```python
from build123d import *

# Parameters (mm, degrees)
PAD_DEPTH       = 10
SKETCH001_W     = 14
SKETCH001_H     = 120
POCKET_DEPTH    = 2
SKETCH002_W     = 8
SKETCH002_H     = 112
POCKET001_DEPTH = 5
SKETCH003_W     = 23
SKETCH003_H     = 6
POCKET002_DEPTH = 2
SKETCH004_R     = 2
POCKET003_DEPTH = 8.001
FILLET_R        = 1
FILLET001_R     = 4
FILLET002_R     = 1
CHAMFER_SIZE    = 1.99
FILLET003_R     = 2
FILLET004_R     = 2
POCKET004_DEPTH = 6.001
SKETCH006_R     = 1.6
POCKET005_DEPTH = 4.5


with BuildPart() as part:
    # Sketch → Pad (new body)
    with BuildSketch(Plane.XY):
        Polygon((0, 6), (20, 6), (20, 126), (34, 126), (34, 6), (42, 6), (42, 0), (20, 0), (20, 4.4), (0, 4.4), align=None)
    extrude(amount=PAD_DEPTH)

    # Sketch001 (on DatumPlane) → Pocket (cut)
    with BuildSketch(Plane.XY.offset(10)):
        with Locations((27, 66)):
            Rectangle(SKETCH001_W, SKETCH001_H)
    extrude(amount=-POCKET_DEPTH, mode=Mode.SUBTRACT)

    # Sketch002 (on DatumPlane) → Pocket001 (cut)
    with BuildSketch(Plane.XY.offset(8)):
        with Locations((27, 62)):
            Rectangle(SKETCH002_W, SKETCH002_H)
    extrude(amount=-POCKET001_DEPTH, mode=Mode.SUBTRACT)

    # Sketch003 (on DatumPlane) → Pocket002 (cut)
    with BuildSketch(Plane.XY.offset(10)):
        with Locations((30.5, 3)):
            Rectangle(SKETCH003_W, SKETCH003_H)
    extrude(amount=-POCKET002_DEPTH, mode=Mode.SUBTRACT)

    # Sketch004 (on DatumPlane) → Pocket003 (cut, through all)
    with BuildSketch(Plane.XY.offset(8)):
        with Locations((27, 122)):
            Circle(SKETCH004_R)
    extrude(amount=-POCKET003_DEPTH, mode=Mode.SUBTRACT)

    # Fillet
    fillet_edges = [part.edges().sort_by_distance(p)[0] for p in [
        (27, 118, 3),
        (31, 62, 3),
        (27, 6, 3),
        (23, 62, 3),
    ]]
    fillet(fillet_edges, radius=FILLET_R)

    # Fillet001
    fillet001_edges = [part.edges().sort_by_distance(p)[0] for p in [
        (20, 126, 4),
        (34, 126, 4),
    ]]
    fillet(fillet001_edges, radius=FILLET001_R)

    # Fillet002
    fillet002_edges = [part.edges().sort_by_distance(p)[0] for p in [
        (20, 64, 8),
        (34, 64, 8),
        (34, 64, 0),
        (20, 64, 0),
    ]]
    fillet(fillet002_edges, radius=FILLET002_R)

    # Chamfer
    chamfer_edges = [part.edges().sort_by_distance(p)[0] for p in [
        (19, 5.2, 10),
    ]]
    chamfer(chamfer_edges, length=CHAMFER_SIZE)

    # Fillet003
    fillet003_edges = [part.edges().sort_by_distance(p)[0] for p in [
        (20, 0, 4),
        (42, 0, 4),
    ]]
    fillet(fillet003_edges, radius=FILLET003_R)

    # Fillet004
    fillet004_edges = [part.edges().sort_by_distance(p)[0] for p in [
        (20, 4.4, 4),
    ]]
    fillet(fillet004_edges, radius=FILLET004_R)

    # Sketch005 (on DatumPlane) → Pocket004 (cut, through all)
    with BuildSketch(Plane(origin=(0, 6, 0), x_dir=(-1, 0, 0), z_dir=(0, 1, 0))):
        Polygon((-3.3, 10), (-2.1, 10), (-2.4, 6), (-3, 6), align=None)
        Polygon((-8.3, 10), (-6.3, 10), (-6.5, 6), (-8.1, 6), align=None)
    extrude(amount=-POCKET004_DEPTH, mode=Mode.SUBTRACT)

    # Sketch006 (on DatumPlane) → Pocket005 (cut)
    with BuildSketch(Plane.YZ.offset(42)):
        with Locations((4.4, 4)):
            Circle(SKETCH006_R)
    extrude(amount=-POCKET005_DEPTH, mode=Mode.SUBTRACT)


solid = part.part
```
The listing builds one solid part. Answer for the finished solid, in the listing's coordinates (mm). A direction names the side the tool comes from. Give positions to 0.01 mm unless a question says otherwise; leave off trailing zeros. Write each loop counter-clockwise with the first axis right and the second up, starting at its lowest first coordinate (ties: lowest second). Pieces come first, ordered by that corner, then holes. Notation, with made-up numbers: (-26, 0.5) -> (5, 0.5) arc R28 cw to (5, 36.5) -> close; hole circle Ø1 at (10.5, -35). An arc over 180 degrees is marked (long way). Write item = value, one per line. Start each with the question number.
1) The part is cut by section A-A, the plane x = 27. Determine the outline of the cut face in (y, z).
2) Straight lines are drawn through the part: line 1 along X through (y, z) = (101, 6.75); line 2 along Z through (x, y) = (39.8, 4.4); line 3 along Y through (x, z) = (6, 7.5). For each, find the intervals that lie inside material, in ascending order.
3) Determine the mould class of faces 4 (the face through (37.5, 4, 4)), 5 (the face through (27, 126, 4)), 6 (the face through (24, 58, 0)) for opening direction Z: +Z half, -Z half, draft (parallel to the pull), parting line (faces both ways), or undercut.
4) Each of these flat-tipped pins is pushed along its axis until it touches: pin 1 (18.5 mm diameter, centred on x = 25.5, y = 59.5, fed in from +Z); pin 2 (1 mm diameter, centred on y = 16, z = 2.5, fed in from +X); pin 3 (1.8 mm diameter, centred on x = 7.5, y = 5.5, fed in from +Z); pin 4 (2 mm diameter, centred on y = 49.5, z = 8, fed in from -X). Where does it stop, or does it pass through?
5) The part is cut by section C-C, the plane x = 36. Determine the outline of the cut face in (y, z).
6) Which of the six approach directions +Z, -Z, +X, -X, +Y, -Y give full straight-line access (tool end or side, diameter ignored) to faces 1 (the face through (27, 118, 6)), 2 (the face through (34, 65, 4)), 3 (the face through (9, 4.4, 5))?
7) The part is cut by section B-B, the plane y = 18.5. Determine the outline of the cut face in (x, z).
Solutions:
q1.outline = (0, 0) -> (120, 0) -> (120, 8) -> (118, 8) -> (118, 4) arc R1 cw to (117, 3) -> (7, 3) arc R1 cw to (6, 4) -> (6, 8) -> (0, 8) -> close; (124, 0) -> (125, 0) arc R1 ccw to (126, 1) -> (126, 7) arc R1 ccw to (125, 8) -> (124, 8) -> close
q2.line_1 = 20 to 23, 31 to 34
q2.line_2 = 0 to 2.4, 5.6 to 8
q2.line_3 = 4.4 to 6
q3.face_4 = undercut
q3.face_5 = draft
q3.face_6 = -Z half
q4.pin_1 = 8
q4.pin_2 = 34
q4.pin_3 = 10
q4.pin_4 = 20
q5.outline = (0, 0) -> (6, 0) -> (6, 8) -> (0, 8) -> close
q6.face_1 = +Z
q6.face_2 = +Z, -Z, +X, +Y
q6.face_3 = +Z, -Z, -X, -Y
q7.outline = (20, 1) arc R1 ccw to (21, 0) -> (33, 0) arc R1 ccw to (34, 1) -> (34, 7) arc R1 ccw to (33, 8) -> (31, 8) -> (31, 4) arc R1 cw to (30, 3) -> (24, 3) arc R1 cw to (23, 4) -> (23, 8) -> (21, 8) arc R1 ccw to (20, 7) -> close
